Here's how the part is built. I have some questions about the finished solid (model axes, mm). Face numbers are marked on the shaded views. Coordinates: 2 decimals unless noted, no trailing zeros. Write each loop counter-clockwise with the first axis right and the second up, starting at its lowest first coordinate (ties: lowest second). Pieces come first, ordered by that corner, then holes. Notation, with made-up numbers: M 5,27 L 28,27 A16 cw 28,32 Z; hole C 13.5,86.25 d2. An arc over 180 degrees is marked long. Use one line per item in the form item = value. Start each with the question number.
1. Please list where these lines run through material, in increasing order: line 1 along X through (y, z) = (3, -4); line 2 along X through (y, z) = (5.5, -2); line 3 along Y through (x, z) = (129, -16). Write a range as [from, to].
2. I'm going to push flat-ended pins straight in: pin 1 Ø4 at (x, z) = (164, -2) entering from -Y; pin 2 Ø2 at (x, y) = (59.5, 5) entering from +Z; pin 3 Ø1 at (y, z) = (3, -15) entering from -X; pin 4 Ø3.5 at (y, z) = (7, -6) entering from +X. Where does each tip first touch, or does it pass through?
3. I want a section at A-A, the plane x = 46. List the corners of the cut face in (y, z) for me.
4. Thinking about a two-plate mould opening in X: for the marked faces 1 and 2, which applies, released by +X, released by -X, zero draft, split by the parting line, or undercut?
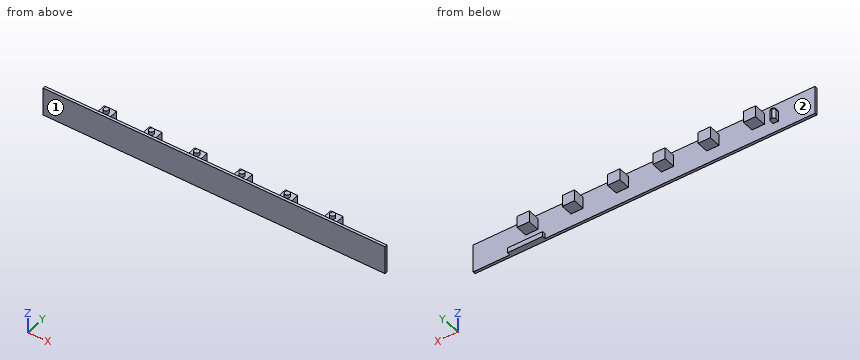
from build123d import *

# Parameters (mm, degrees)
SKETCH1_W           = 204
SKETCH1_H           = 17
BOSS_EXTRUDE1_DEPTH = 1.6
SKETCH2_W           = 7.3
SKETCH2_H           = 6.9
BOSS_EXTRUDE2_DEPTH = 7.1
SKETCH6_R           = 1.5
BOSS_EXTRUDE6_DEPTH = 2.1
SKETCH4_W           = 3.3
SKETCH4_H           = 7.2
BOSS_EXTRUDE4_DEPTH = 3.6
SKETCH5_W           = 21
SKETCH5_H           = 3
BOSS_EXTRUDE5_DEPTH = 2
LPATTERN1_COUNT     = 6
LPATTERN1_PITCH     = 27
FILLET1_R           = 1.5


with BuildPart() as part:
    # Sketch1 → Boss-Extrude1 (new body)
    with BuildSketch(Plane(origin=(0, 0, 0), x_dir=(1, 0, 0), z_dir=(0, 1, 0))):
        with Locations((102, 8.5)):
            Rectangle(SKETCH1_W, SKETCH1_H)
    extrude(amount=BOSS_EXTRUDE1_DEPTH)

    # Sketch2 → Boss-Extrude2 (add)
    with BuildSketch(Plane(origin=(0, 1.6, 0), x_dir=(1, 0, 0), z_dir=(0, 1, 0))):
        with Locations((33.95, 5.65)):
            Rectangle(SKETCH2_W, SKETCH2_H)
    boss_extrude2 = extrude(amount=BOSS_EXTRUDE2_DEPTH)

    # Sketch6 → Boss-Extrude6 (add)
    with BuildSketch(Plane.XY.offset(-2.2)):
        with Locations(Location((33.95, 5.15, 0), (0, 0, 180))):
            Circle(SKETCH6_R)
    boss_extrude6 = extrude(amount=BOSS_EXTRUDE6_DEPTH)

    # Sketch4 → Boss-Extrude4 (add)
    with BuildSketch(Plane(origin=(0, 1.6, 0), x_dir=(1, 0, 0), z_dir=(0, 1, 0))):
        with Locations((23.350594588, 7.718433613)):
            Rectangle(SKETCH4_W, SKETCH4_H)
    extrude(amount=BOSS_EXTRUDE4_DEPTH)

    # Sketch5 → Boss-Extrude5 (add)
    with BuildSketch(Plane(origin=(0, 1.6, 0), x_dir=(1, 0, 0), z_dir=(0, 1, 0))):
        with Locations((171.5, 15.5)):
            Rectangle(SKETCH5_W, SKETCH5_H)
    extrude(amount=BOSS_EXTRUDE5_DEPTH)

    # LPattern1: Boss-Extrude2, Boss-Extrude6 ×6
    with Locations(*[(i * LPATTERN1_PITCH, 0, 0) for i in range(1, LPATTERN1_COUNT)]):
        add(boss_extrude2)
        add(boss_extrude6)

    # Fillet1
    fillet1_edges = [part.edges().sort_by_distance(p)[0] for p in [
        (21.700594588, 3.4, -4.118433613),
        (25.000594588, 3.4, -4.118433613),
        (21.700594588, 5.2, -7.718433613),
        (23.350594588, 5.2, -4.118433613),
        (25.000594588, 5.2, -7.718433613),
    ]]
    fillet(fillet1_edges, radius=FILLET1_R)


solid = part.part
Answer list:
q1.line_1 = [30.3, 37.6], [57.3, 64.6], [84.3, 91.6], [111.3, 118.6], [138.3, 145.6], [165.3, 172.6]
q1.line_2 = [32.49, 35.41], [59.49, 62.41], [86.49, 89.41], [113.49, 116.41], [140.49, 143.41], [167.49, 170.41]
q1.line_3 = [0, 1.6]
q2.pin_1 = 0
q2.pin_2 = -0.1
q2.pin_3 = 161
q2.pin_4 = 172.6
q3.outline = M 0,-17 L 1.6,-17 L 1.6,0 L 0,0 Z
q4.face_1 = zero draft
q4.face_2 = undercut
